Geometry check sheet. Reference: the model listing, model coordinates, mm. A direction names the side the tool comes from. Coordinates: 2 decimals unless noted, no trailing zeros. Write each loop counter-clockwise with the first axis right and the second up, starting at its lowest first coordinate (ties: lowest second). Pieces come first, ordered by that corner, then holes. Notation, with made-up numbers: (14, -8.5) -> (44, -8.5) arc R8 ccw to (44, 3.5) -> close; hole circle Ø8 at (-18, 9). An arc over 180 degrees is marked (long way). Answer as CSV lines item,"result".
Autodesk Inventor part; units mm, degrees
ref_plane "YZ Plane" through (0, 0, 0) normal (1, 0, 0) x (0, 1, 0)
ref_plane "XZ Plane" through (0, 0, 0) normal (0, 1, 0) x (-1, 0, 0)
ref_plane "XY Plane" through (0, 0, 0) normal (0, 0, 1) x (1, 0, 0)
sketch "Sketch1" plane through (0, 0, 0) normal (0, 0, 1) x (1, 0, 0)
  line L0 (0, 0) -> (330, 0)
  line L1 (330, 0) -> (330, 510)
  line L2 (330, 510) -> (0, 510)
  line L3 (0, 510) -> (0, 0)
  dimension "d0" = 330
  dimension "d1" = 510
extrude "Extrusion1" add sketch "Sketch1" along normal blind 150
sketch "Sketch2" plane through (0, 0, 0) normal (0, -1, 0) x (1, 0, 0)
  circle A0 centre (165, -304.672) radius 315
  line L0 (85, 0) -> (245, 0)
  line L1 (0, 0) -> (330, 0)
  circle A1 centre (165, -304.672) radius 317
  point P0 (165, 0)
  point P1 (165, 0)
  dimension "d4" = 630
  dimension "d8" = 160
  dimension "d9" = 2
extrude "Extrusion2" cut sketch "Sketch2" against normal through all
sketch "Sketch3" plane through (0, 0, 150) normal (0, 0, 1) x (1, 0, 0)
  line L0 (0, 0) -> (330, 0)
  line L1 (330, 0) -> (330, 510)
  line L2 (330, 510) -> (0, 510)
  line L3 (0, 510) -> (0, 0)
  line L4 (10, 10) -> (320, 10)
  line L5 (320, 10) -> (320, 500)
  line L6 (320, 500) -> (10, 500)
  line L7 (10, 500) -> (10, 10)
  dimension "d10" = 10
extrude "Extrusion3" cut sketch "Sketch3" against normal blind 130 contours L7 L6 L5 L4
sketch "Sketch4" plane through (0, 0, 20) normal (0, 0, 1) x (1, 0, 0)
  line L0 (10, 500) -> (320, 500) construction
  line L1 (85, 500) -> (245, 500) construction
  line L2 (245, 500) -> (245, 10) construction
  line L3 (245, 10) -> (85, 10) construction
  line L4 (85, 10) -> (85, 500) construction
  line L5 (320, 10) -> (10, 10) construction
  line L6 (85, 500) -> (245, 500) construction
  line L7 (245, 500) -> (245, 455) construction
  line L8 (245, 455) -> (85, 455) construction
  line L9 (85, 455) -> (85, 500) construction
  line L10 (85, 455) -> (245, 455) construction
  line L11 (245, 455) -> (245, 400) construction
  line L12 (245, 400) -> (85, 400) construction
  line L13 (85, 400) -> (85, 455) construction
  line L14 (85, 400) -> (245, 400) construction
  line L15 (245, 400) -> (245, 345) construction
  line L16 (245, 345) -> (85, 345) construction
  line L17 (85, 345) -> (85, 400) construction
  line L18 (85, 345) -> (245, 345) construction
  line L19 (245, 345) -> (245, 290) construction
  line L20 (245, 290) -> (85, 290) construction
  line L21 (85, 290) -> (85, 345) construction
  line L22 (85, 290) -> (245, 290) construction
  line L23 (245, 290) -> (245, 235) construction
  line L24 (245, 235) -> (85, 235) construction
  line L25 (85, 235) -> (85, 290) construction
  circle A0 centre (130.3559, 262.5) radius 15
  circle A1 centre (199.6441, 262.5) radius 15
  line L26 (130.3559, 262.5) -> (199.6441, 262.5) construction
  point P0 (0, 0)
  point P1 (165, 500)
  point P2 (165, 500)
  point P3 (165, 262.5)
  point P4 (165, 235)
  point P5 (245, 262.5)
  dimension "d13" = 160
  dimension "d14" = 45
  dimension "d15" = 55
  dimension "d16" = 55
  dimension "d17" = 55
  dimension "d18" = 55
  dimension "d19" = 30
  dimension "d20" = 30
  dimension "d21" = 69.2883
extrude "Extrusion4" cut sketch "Sketch4" against normal through all
sketch "Sketch5" plane through (0, 0, 150) normal (0, 0, 1) x (1, 0, 0)
  line L0 (0, 0) -> (330, 0)
  line L1 (77.4557, 510) -> (252.5443, 510)
  line L2 (0, 0) -> (165, 0)
  line L3 (165, 0) -> (165, 510)
  line L4 (165, 510) -> (0, 510)
  line L5 (0, 510) -> (0, 0)
  line L6 (330, 0) -> (330, 510)
  line L7 (0, 0) -> (330, 0)
  line L8 (330, 0) -> (330, 340)
  line L9 (330, 340) -> (0, 340)
  line L10 (0, 340) -> (0, 0)
  dimension "d24" = 340
extrude "Extrusion5" cut sketch "Sketch5" against normal through all
properties part number "CA002" material "ABS Plastic"
Item 1: Cross-section at C-C, the plane y = 423.5. Record the cut outline in (x, z), plus the area to 3 significant figures.
Responses:
outline,"(165, 12.33) arc R317 cw to (252.54, 0) -> (330, 0) -> (330, 150) -> (320, 150) -> (320, 20) -> (165, 20) -> close"
area,"3,880 mm2"
Item 2: Set-up check for faces 1 (the flat face through (249, 510, 74)), 2 (the flat face through (244, 500, 86)): record each of +Z, -Z, +X, -X, +Y, -Y from which the full face is reachable in a straight line by a thin tool's end or side.
Responses:
face 1,"+Z, -Z, +X, -X, +Y"
face 2,"+Z, -X, -Y"
Item 3: Cross-section at A-A, the plane x = 296. Record the cut outline in (y, z).
Responses:
outline,"(340, 0) -> (510, 0) -> (510, 150) -> (500, 150) -> (500, 20) -> (340, 20) -> close"
Item 4: Depth check by flat-ended pin: pin 1 Ø1 at (x, z) = (270.5, 32) entering from -Y; pin 2 Ø1 at (x, y) = (227.5, 417) entering from +Z; pin 3 Ø1.5 at (y, z) = (389.5, 131.5) entering from -X. Enter the tip coordinate at first touch or a pass-through.
Responses:
pin 1,"stops at y = 500"
pin 2,"stops at z = 20"
pin 3,"stops at x = 320"
Item 5: Cross-section at B-B, the plane z = 94. Record the cut outline in (x, y).
Responses:
outline,"(165, 500) -> (320, 500) -> (320, 340) -> (330, 340) -> (330, 510) -> (165, 510) -> close"
Item 6: Thickness scan on probe 1 along X at (y, z) = (497, 140.5); probe 2 along Y at (x, z) = (220, 142); probe 3 along Z at (x, y) = (302, 389.5). Record the ranges inside material, lowest first.
Responses:
probe 1,"x = 320 to 330"
probe 2,"y = 500 to 510"
probe 3,"z = 0 to 20"
